The drawing under review shows one solid part. Ordinate dimensions are in mm from its lowest x, y, z. A direction names the side the tool comes from. Give positions to 0.01 mm unless a question says otherwise; leave off trailing zeros. Order: outer loops, then holes, each group sorted by start corner. A loop starts at its lowest first (then second) coordinate and runs counter-clockwise, first axis right, second up. Notation, with made-up numbers: M 60,65 L 98,65 A27 ccw 98,98 Z; hole C -22.75,3.5 d10. An arc over 180 degrees is marked long. Put each result on its own line as item: value. Start each with the question number.
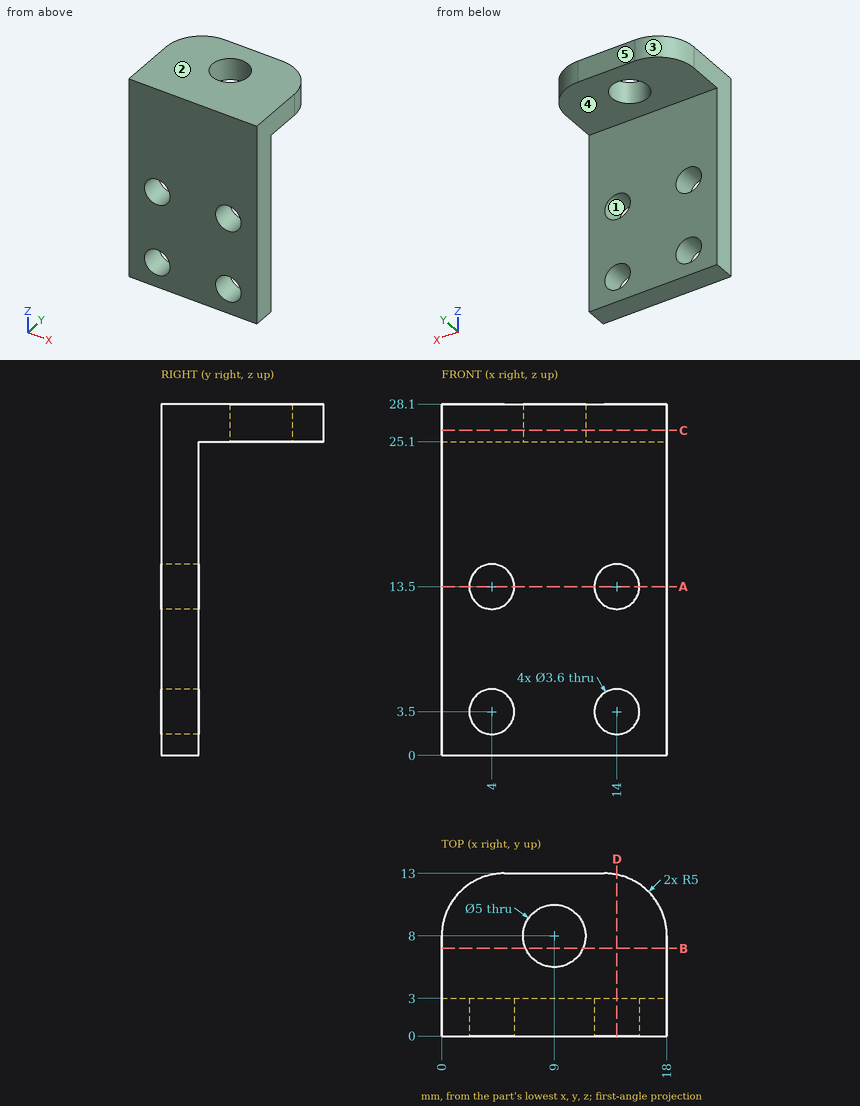
1. To check wall thickness, follow probe 1 along Z at (x, y) = (14, 1.65); probe 2 along X at (y, z) = (2, 3.5); probe 3 along Z at (x, y) = (12.5, 1). State the ranges of each line that lie inside material, in increasing order.
2. Machinability: for the marked faces 4 and 5, which of the approach directions +Z, -Z, +X, -X, +Y, -Y give a long, thin tool a straight path to every point of the face, cutting with its end or side? Answer none if there is none.
3. Consider section D-D on x = 14. Give the boundary of the cut face in (y, z), then the cut area to 3 significant figures.
4. Consider section C-C on z = 26. Give the boundary of the cut face in (x, y).
5. The part is to be moulded in two halves that separate along Z. For the marked faces 1, 2 and 3, say which applies: +Z half, -Z half, draft (parallel to the pull), parting line (faces both ways), or undercut.
6. Insertion check: pin 1 (2 mm diameter, centred on x = 14, z = 3.5, fed in from +Y); pin 2 (5 mm diameter, centred on x = 3.5, y = 10.5, fed in from -Z); pin 3 (4.5 mm diameter, centred on x = 14, z = 13.5, fed in from +Y). Each pin has a flat end and moves straight along its axis. Give the tip position at first contact, or say it passes through.
7. Consider section B-B on y = 7. Give the boundary of the cut face in (x, z), then the cut area to 3 significant figures.
8. Consider section A-A on z = 13.5. Give the boundary of the cut face in (x, y).
Returned:
1. probe 1: z = 0 to 1.7, 5.3 to 11.7, 15.3 to 28.1
1. probe 2: x = 0 to 2.2, 5.8 to 12.2, 15.8 to 18
1. probe 3: z = 0 to 2.51, 4.49 to 12.51, 14.49 to 28.1
2. face 4: -Z, +X, -X, +Y
2. face 5: +Z, -Z, +X, -X, +Y
3. outline: M 0,0 L 3,0 L 3,1.7 L 0,1.7 Z; M 0,5.3 L 3,5.3 L 3,11.7 L 0,11.7 Z; M 0,15.3 L 3,15.3 L 3,25.1 L 12.9,25.1 L 12.9,28.1 L 0,28.1 Z
3. area: 92.4 mm2
4. outline: M 0,0 L 18,0 L 18,8 A5 ccw 13,13 L 5,13 A5 ccw 0,8 Z; hole C 9,8 d5
5. face 1: undercut
5. face 2: +Z half
5. face 3: draft
6. pin 1: passes through
6. pin 2: stops at z = 25.1
6. pin 3: stops at y = 3
7. outline: M 0,25.1 L 6.71,25.1 L 6.71,28.1 L 0,28.1 Z; M 11.29,25.1 L 18,25.1 L 18,28.1 L 11.29,28.1 Z
7. area: 40.3 mm2
8. outline: M 0,0 L 2.2,0 L 2.2,3 L 0,3 Z; M 5.8,0 L 12.2,0 L 12.2,3 L 5.8,3 Z; M 15.8,0 L 18,0 L 18,3 L 15.8,3 Z
